For this review, take the finished solid that the model builds, in its own axes (mm). A direction names the side the tool comes from. Round coordinates to 2 decimals unless told otherwise and drop trailing zeros. Write each loop counter-clockwise with the first axis right and the second up, starting at its lowest first coordinate (ties: lowest second). Pieces come first, ordered by that corner, then holes. Notation, with made-up numbers: M -31.5,-4 L -21.5,-4 A19 ccw -21.5,33 Z; hole C 88.25,76 d2. An arc over 180 degrees is marked long. Use one line per item in the form item = value. Start each with the question number.
Item 1: Add section B-B (x = 0). State the section outline as (y, z) points.
Item 2: Add section C-C (x = 23.5). Count the separate pieces of the cut face and the enclosed holes in it, and give its area (3 significant figures).
Item 3: For faces 1 (the cylindrical face through (-9.67, -10.34, 24.48)), 2 (the flat face through (-26.83, 33.9, 31.94)), 3 (the cylindrical face through (27.52, -27.62, 28.85)), list the 3-axis set-ups (+Z, -Z, +X, -X, +Y, -Y) from which the entire face can be reached by the end or side of a thin tool; tool diameter is ignored.
Item 4: Draft analysis for pull direction X (two halves, no side actions). For faces 4 (the flat face through (-32, 32, 51)), 5 (the flat face through (-11, -1, 26)), 6 (the cylindrical face through (51.997, -0.572, 24.479)), state which applies: released by +X, released by -X, zero draft, split by the parting line, or undercut.
Item 5: For line 1 (Y direction, x = -33, z = 44.5); line 2 (Z direction, x = -28.5, y = -40.5); line 3 (Y direction, x = 32, z = 37), list the stretches that pass through material, from the lowest coordinate up. Write a range as [from, to].
Item 6: For P1, Ø1.5, axis at x = 33, y = -33, coming from the +Z side; P2, Ø8, axis at y = -37.5, z = 44.5, coming from the -X side; P3, Ø8, axis at y = 24, z = 28, coming from the -X side, all flat-tipped, find the tip position at first contact; note any pin that passes through.
Item 7: Add section D-D (y = 12). State the section outline as (x, z) points.
from build123d import *

# Parameters (mm, degrees)
SKETCH003_R             = 52
SKETCH003_R_2           = 1.6
SKETCH003_R_3           = 2.2
PAD002_DEPTH            = 3
SKETCH005_R             = 5
PAD004_DEPTH            = 28
SKETCH007_R             = 1.5
POCKET002_DEPTH         = 10
SKETCH011_R             = 1.8
POCKET004_DEPTH         = 5
PAD011_DEPTH            = 5
PAD012_DEPTH            = 5
BODY001_PLACEMENT_ANGLE = 180


with BuildPart() as part:
    # Sketch003 → Pad002 (new body)
    with BuildSketch(Plane.XY):
        Circle(SKETCH003_R)
        Circle(SKETCH003_R_2, mode=Mode.SUBTRACT)
        with Locations((8.485281, 8.485281)):
            Circle(SKETCH003_R_3, mode=Mode.SUBTRACT)
        with Locations((-8.485281, 8.485281)):
            Circle(SKETCH003_R_3, mode=Mode.SUBTRACT)
        with Locations((-8.485281, -8.485281)):
            Circle(SKETCH003_R_3, mode=Mode.SUBTRACT)
        with Locations((8.485281, -8.485281)):
            Circle(SKETCH003_R_3, mode=Mode.SUBTRACT)
    extrude(amount=PAD002_DEPTH)

    # Sketch005 → Pad004 (join)
    with BuildSketch(Plane.XY):
        with Locations((33.234019, 33.234019)):
            Circle(SKETCH005_R)
        with Locations((-33.234019, 33.234019)):
            Circle(SKETCH005_R)
        with Locations((-33.234019, -33.234019)):
            Circle(SKETCH005_R)
        with Locations((33.234019, -33.234019)):
            Circle(SKETCH005_R)
    extrude(amount=PAD004_DEPTH)

    # Sketch007 → Pocket002 (cut)
    with BuildSketch(Plane.XY.offset(28)):
        with Locations((33.234019, 33.234019)):
            Circle(SKETCH007_R)
        with Locations((-33.234019, 33.234019)):
            Circle(SKETCH007_R)
        with Locations((-33.234019, -33.234019)):
            Circle(SKETCH007_R)
        with Locations((33.234019, -33.234019)):
            Circle(SKETCH007_R)
    extrude(amount=-POCKET002_DEPTH, mode=Mode.SUBTRACT)

    # Sketch011 → Pocket004 (cut)
    with BuildSketch(Plane.XY):
        with Locations((23.5, 40.703194)):
            Circle(SKETCH011_R)
        with Locations((-40.703194, 23.5)):
            Circle(SKETCH011_R)
        with Locations((-23.5, -40.703194)):
            Circle(SKETCH011_R)
        with Locations((40.703194, -23.5)):
            Circle(SKETCH011_R)
        with Locations((-23.5, 40.703194)):
            Circle(SKETCH011_R)
        with Locations((40.703194, 23.5)):
            Circle(SKETCH011_R)
        with Locations((23.5, -40.703194)):
            Circle(SKETCH011_R)
        with Locations((-40.703194, -23.5)):
            Circle(SKETCH011_R)
    extrude(amount=POCKET004_DEPTH, mode=Mode.SUBTRACT)

    # Sketch018 → Pad011 (join, symmetric)
    with BuildSketch(Plane(origin=(0, 0, 0), x_dir=(-0.707107, 0.707107, 0), z_dir=(0.707107, 0.707107, 0))):
        with BuildLine():
            Line((-47, 18), (-47, 3))
            Line((-47, 3), (-32, 3))
            ThreePointArc((-42, 13), (-39.071068, 5.928932), (-32, 3))
            Line((-42, 13), (-42, 18))
            Line((-42, 18), (-47, 18))
        make_face()
        with BuildLine():
            Line((47, 18), (47, 3))
            Line((47, 3), (32, 3))
            ThreePointArc((32, 3), (39.071068, 5.928932), (42, 13))
            Line((42, 13), (42, 18))
            Line((42, 18), (47, 18))
        make_face()
    extrude(amount=PAD011_DEPTH, both=True)

    # Sketch019 → Pad012 (join, symmetric)
    with BuildSketch(Plane(origin=(0, 0, 0), x_dir=(0.707107, 0.707107, 0), z_dir=(0.707107, -0.707107, 0))):
        with BuildLine():
            Line((-47, 18), (-47, 3))
            Line((-47, 3), (-32, 3))
            ThreePointArc((-42, 13), (-39.071068, 5.928932), (-32, 3))
            Line((-42, 13), (-42, 18))
            Line((-42, 18), (-47, 18))
        make_face()
        with BuildLine():
            Line((47, 18), (47, 3))
            Line((47, 3), (32, 3))
            ThreePointArc((32, 3), (39.071068, 5.928932), (42, 13))
            Line((42, 13), (42, 18))
            Line((42, 18), (47, 18))
        make_face()
    extrude(amount=PAD012_DEPTH, both=True)


with BuildPart() as part_1:
    # Body001 placement: moved
    add(part.part.moved(Location((0, 0, 23))).rotate(Axis((0, 0, 23), (0, 0, -1)), BODY001_PLACEMENT_ANGLE))


solid = part_1.part
Calculated:
q1.outline = M -52,23 L -1.6,23 L -1.6,26 L -52,26 Z; M 1.6,23 L 52,23 L 52,26 L 1.6,26 Z
q2.separate_pieces = 3
q2.enclosed_holes = 0
q2.area = 269 mm^2
q3.face_1 = +Z, -Z
q3.face_2 = +Z, +Y
q3.face_3 = +Z
q4.face_4 = zero draft
q4.face_5 = undercut
q4.face_6 = released by +X
q5.line_1 = [-38.23, -34.72], [-31.75, -28.24], [28.24, 31.75], [34.72, 38.23]
q5.line_2 = [23, 26]
q5.line_3 = [-38.08, -27.4], [27.4, 38.08]
q6.P1 = 41
q6.P2 = -38.23
q6.P3 = -47.77
q7.outline = M -50.6,23 L 50.6,23 L 50.6,26 L -50.6,26 Z
